```python
from build123d import *

# Parameters (mm, degrees)
SKETCH1_W           = 103.5
SKETCH1_H           = 66
BOSS_EXTRUDE1_DEPTH = 1.6
SKETCH3_R           = 1.3
CUT_EXTRUDE2_DEPTH  = 10
CUT_EXTRUDE3_REACH  = 63.397
SKETCH4_R           = 1.75


with BuildPart() as part:
    # Sketch1 → Boss-Extrude1 (new body)
    with BuildSketch(Plane(origin=(0, 0, 0), x_dir=(1, 0, 0), z_dir=(0, 1, 0))):
        Rectangle(SKETCH1_W, SKETCH1_H)
    extrude(amount=BOSS_EXTRUDE1_DEPTH)

    # Sketch3 → Cut-Extrude2 (cut)
    with BuildSketch(Plane(origin=(0, 1.6, 0), x_dir=(1, 0, 0), z_dir=(0, 1, 0))):
        with Locations(Location((-33.052335, 28, 0), (0, 0, 270))):
            Circle(SKETCH3_R)
        with Locations(Location((-33.052335, -28, 0), (0, 0, 270))):
            Circle(SKETCH3_R)
    extrude(amount=-CUT_EXTRUDE2_DEPTH, mode=Mode.SUBTRACT)

    # Sketch4 → Cut-Extrude3 (cut, up to next)
    with BuildSketch(Plane(origin=(0, 1.6, 0), x_dir=(1, 0, 0), z_dir=(0, 1, 0)), mode=Mode.PRIVATE) as cut_extrude3_sk1:
        with Locations(Location((24.75, 25, 0), (0, 0, 270))):
            Circle(SKETCH4_R)
    cut_extrude3_tool1 = extrude(cut_extrude3_sk1.sketch, amount=-CUT_EXTRUDE3_REACH, mode=Mode.PRIVATE) & part.part
    # Sketch4 → Cut-Extrude3 (cut, up to next)
    with BuildSketch(Plane(origin=(0, 1.6, 0), x_dir=(1, 0, 0), z_dir=(0, 1, 0)), mode=Mode.PRIVATE) as cut_extrude3_sk2:
        with Locations(Location((24.75, -25, 0), (0, 0, 270))):
            Circle(SKETCH4_R)
    cut_extrude3_tool2 = extrude(cut_extrude3_sk2.sketch, amount=-CUT_EXTRUDE3_REACH, mode=Mode.PRIVATE) & part.part
    add(cut_extrude3_tool1.solids().sort_by_distance((24.75, 1.6, -25))[0], mode=Mode.SUBTRACT)
    add(cut_extrude3_tool2.solids().sort_by_distance((24.75, 1.6, 25))[0], mode=Mode.SUBTRACT)


solid = part.part
```
Design review of the part built by this model. Coordinates are the model's own, in mm. Give positions to 0.01 mm unless a question says otherwise; leave off trailing zeros. Loops run counter-clockwise (first coordinate to the right, second up) from the corner with the lowest first, then second, coordinate; pieces in that order, holes last. Notation, with made-up numbers: (6, 63) -> (22, 63) arc R26 cw to (22, 87) -> close; hole circle Ø7 at (2.5, -36.5). An arc over 180 degrees is marked (long way). Write each question's results on one line, items separated by ' | '.
Q1. Take a section at B-B, the plane z = 25. Write out the cut boundary in (x, y), plus the area to 3 significant figures.
Reply:
outline: (-51.75, 0) -> (23, 0) -> (23, 1.6) -> (-51.75, 1.6) -> close; (26.5, 0) -> (51.75, 0) -> (51.75, 1.6) -> (26.5, 1.6) -> close | area: 160 mm²
Q2. Wall thickness on L1, parallel to Z at x = 25, y = 0.75; L2, parallel to X at y = 0.9, z = -28; L3, parallel to X at y = 1.5, z = -29: over which ranges is each line inside the solid? List them lowest first.
Reply:
L1: z = -33 to -26.73, -23.27 to 23.27, 26.73 to 33 | L2: x = -51.75 to -34.35, -31.75 to 51.75 | L3: x = -51.75 to -33.88, -32.22 to 51.75
Q3. Take a section at A-A, the plane x = 24.75. Write out the cut boundary in (y, z), plus the area to 3 significant figures.
Reply:
outline: (0, -33) -> (1.6, -33) -> (1.6, -26.75) -> (0, -26.75) -> close; (0, -23.25) -> (1.6, -23.25) -> (1.6, 23.25) -> (0, 23.25) -> close; (0, 26.75) -> (1.6, 26.75) -> (1.6, 33) -> (0, 33) -> close | area: 94.4 mm²
Q4. The part is to be moulded in two halves that separate along X. For faces 1 (the face through (-1, 0, 0)), 2 (the face through (26.485, 0.811, 24.772)), 3 (the face through (25.93, 0.81, -26.29)), say which applies: +X half, -X half, draft (parallel to the pull), parting line (faces both ways), or undercut.
Reply:
face 1: draft | face 2: undercut | face 3: undercut
